Design review of the part built by this model. Coordinates are the model's own, in mm. Face numbers are marked on the shaded views. A direction names the side the tool comes from. Coordinates: 2 decimals unless noted, no trailing zeros. Loops run counter-clockwise (first coordinate to the right, second up) from the corner with the lowest first, then second, coordinate; pieces in that order, holes last. Notation, with made-up numbers: (0, 60.25) -> (59, 60.25) arc R34 ccw to (59, 97.25) -> close; hole circle Ø1 at (78.25, 46.25). An arc over 180 degrees is marked (long way). Use a Markdown table: item, result. Add a question column.
Q1. For the marked faces 1 and 2, list the 3-axis set-ups (+Z, -Z, +X, -X, +Y, -Y) from which the entire face can be reached by the end or side of a thin tool; tool diameter is ignored.
Q2. For probe 1 along X at (y, z) = (1.7, 20.25); probe 2 along Z at (x, y) = (5, -2.7); probe 3 along Z at (x, y) = (4.5, 0.95), list the stretches that pass through material, from the lowest coordinate up.
Q3. Clearance check with flat-ended pins moving along their axes: pin 1 Ø0.9 at (x, z) = (4, 4) entering from -Y; pin 2 Ø2.5 at (x, z) = (5, 12) entering from -Y; pin 3 Ø12 at (x, z) = (15.5, 17.5) entering from +Y. State where each tip first meets the part, or that it passes through.
Q4. Take a section at C-C on z = 12. Write out the cut boundary in (x, y), plus the area to 3 significant figures.
Q5. Take a section at D-D on x = 20. Write out the cut boundary in (y, z).
Q6. Take a section at B-B on z = 3.75. Write out the cut boundary in (x, y), plus the area to 3 significant figures.
Q7. Take a section at A-A on y = 0.75. Write out the cut boundary in (x, z), plus the area to 3 significant figures.
from build123d import *

# Parameters (mm, degrees)
SKETCH1_W           = 50
SKETCH1_H           = 24
BOSS_EXTRUDE1_DEPTH = 3
SKETCH2_R           = 3
SKETCH2_R_2         = 1.5
BOSS_EXTRUDE2_DEPTH = 4
SKETCH3_R           = 0.9
CUT_EXTRUDE1_DEPTH  = 10
SKETCH4_R           = 1.5
SKETCH4_R_2         = 0.75
BOSS_EXTRUDE3_DEPTH = 5
SKETCH5_R           = 1.5
CUT_EXTRUDE2_DEPTH  = 10


with BuildPart() as part:
    # Sketch1 → Boss-Extrude1 (new body)
    with BuildSketch(Plane(origin=(0, 0, 0), x_dir=(1, 0, 0), z_dir=(0, 1, 0))):
        with Locations((25, -12)):
            Rectangle(SKETCH1_W, SKETCH1_H)
    extrude(amount=BOSS_EXTRUDE1_DEPTH)

    # Sketch2 → Boss-Extrude2 (add)
    with BuildSketch(Plane.XZ):
        with Locations((5, 12)):
            Circle(SKETCH2_R)
        with Locations((5, 12)):
            Circle(SKETCH2_R_2, mode=Mode.SUBTRACT)
        with Locations((45, 12)):
            Circle(SKETCH2_R)
        with Locations((45, 12)):
            Circle(SKETCH2_R_2, mode=Mode.SUBTRACT)
    extrude(amount=BOSS_EXTRUDE2_DEPTH)

    # Sketch3 → Cut-Extrude1 (cut)
    with BuildSketch(Plane(origin=(0, 3, 0), x_dir=(1, 0, 0), z_dir=(0, 1, 0))):
        with Locations((4.5, -3.75)):
            Circle(SKETCH3_R)
        with Locations((45.5, -3.75)):
            Circle(SKETCH3_R)
        with Locations((45.5, -20.25)):
            Circle(SKETCH3_R)
        with Locations((4.5, -20.25)):
            Circle(SKETCH3_R)
    extrude(amount=-CUT_EXTRUDE1_DEPTH, mode=Mode.SUBTRACT)

    # Sketch4 → Boss-Extrude3 (add)
    with BuildSketch(Plane(origin=(0, 3, 0), x_dir=(1, 0, 0), z_dir=(0, 1, 0))):
        with Locations((4.5, -3.75)):
            Circle(SKETCH4_R)
        with Locations((4.5, -3.75)):
            Circle(SKETCH4_R_2, mode=Mode.SUBTRACT)
        with Locations((45.5, -3.75)):
            Circle(SKETCH4_R)
        with Locations((45.5, -3.75)):
            Circle(SKETCH4_R_2, mode=Mode.SUBTRACT)
        with Locations((4.5, -20.25)):
            Circle(SKETCH4_R)
        with Locations((4.5, -20.25)):
            Circle(SKETCH4_R_2, mode=Mode.SUBTRACT)
        with Locations((45.5, -20.25)):
            Circle(SKETCH4_R)
        with Locations((45.5, -20.25)):
            Circle(SKETCH4_R_2, mode=Mode.SUBTRACT)
    extrude(amount=BOSS_EXTRUDE3_DEPTH)

    # Sketch5 → Cut-Extrude2 (cut)
    with BuildSketch(Plane.XZ):
        with Locations((5, 12)):
            Circle(SKETCH5_R)
        with Locations((45, 12)):
            Circle(SKETCH5_R)
    extrude(amount=-CUT_EXTRUDE2_DEPTH, mode=Mode.SUBTRACT)


solid = part.part
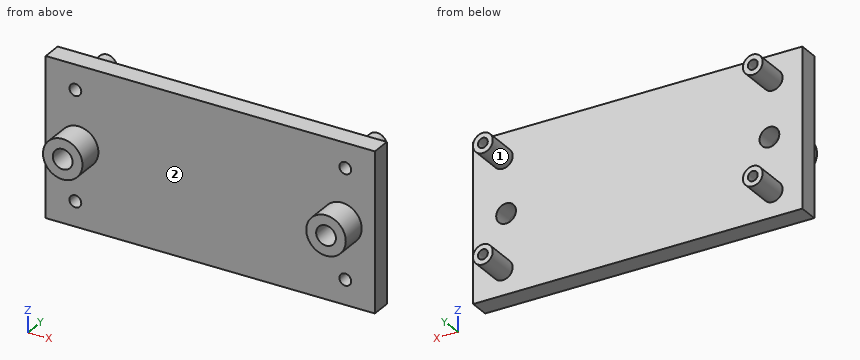
Answer list:
| question | item | result |
|---|---|---|
| 1 | face 1 | +Y |
| 1 | face 2 | -Y |
| 2 | probe 1 | 0 to 3.6, 5.4 to 44.6, 46.4 to 50 |
| 2 | probe 2 | 9 to 10.5, 13.5 to 15 |
| 2 | probe 3 | 0 to 2.85, 4.65 to 10.59, 13.41 to 19.35, 21.15 to 24 |
| 3 | pin 1 | y = 0 |
| 3 | pin 2 | through |
| 3 | pin 3 | y = 3 |
| 4 | outline | (0, 0) -> (2, 0) -> (2, -4) -> (3.5, -4) -> (3.5, 3) -> (0, 3) -> close; (6.5, -4) -> (8, -4) -> (8, 0) -> (42, 0) -> (42, -4) -> (43.5, -4) -> (43.5, 3) -> (6.5, 3) -> close; (46.5, -4) -> (48, -4) -> (48, 0) -> (50, 0) -> (50, 3) -> (46.5, 3) -> close |
| 4 | area | 156 mm² |
| 5 | outline | (0, 0) -> (3, 0) -> (3, 24) -> (0, 24) -> close |
| 6 | outline | (0, 0) -> (3.6, 0) -> (3.6, 3) -> (3.75, 3) -> (3.75, 8) -> (3, 8) -> (3, 3) -> (0, 3) -> close; (5.25, 3) -> (5.4, 3) -> (5.4, 0) -> (44.6, 0) -> (44.6, 3) -> (44.75, 3) -> (44.75, 8) -> (44, 8) -> (44, 3) -> (6, 3) -> (6, 8) -> (5.25, 8) -> close; (46.25, 3) -> (46.4, 3) -> (46.4, 0) -> (50, 0) -> (50, 3) -> (47, 3) -> (47, 8) -> (46.25, 8) -> close |
| 6 | area | 154 mm² |
| 7 | outline | (0, 0) -> (50, 0) -> (50, 24) -> (0, 24) -> close; hole circle Ø3 at (5, 12); hole circle Ø1.8 at (4.5, 3.75); hole circle Ø1.8 at (4.5, 20.25); hole circle Ø3 at (45, 12); hole circle Ø1.8 at (45.5, 3.75); hole circle Ø1.8 at (45.5, 20.25) |
| 7 | area | 1,180 mm² |
